For this review, take the finished solid that the model builds, in its own axes (mm). Face numbers are marked on the shaded views. A direction names the side the tool comes from. Give positions to 0.01 mm unless a question says otherwise; leave off trailing zeros. Order: outer loops, then holes, each group sorted by start corner. A loop starts at its lowest first (then second) coordinate and runs counter-clockwise, first axis right, second up. Notation, with made-up numbers: (-2, 33) - (44, 33) arc R19 ccw to (44, 55) - close; hole circle Ø7 at (-38, 33). An arc over 180 degrees is marked (long way). Use a Markdown table: item, result. Add a question column.
1) Clearance check with flat-ended pins moving along their axes: P1, Ø6, axis at x = 21, z = 28.5, coming from the +Y side; P2, Ø1.2, axis at x = -46.5, z = 11.5, coming from the -Y side; P3, Ø6, axis at x = -24.5, z = 20.5, coming from the -Y side. State where each tip first meets the part, or that it passes through.
2) We need section A-A on z = 31.5. Write out the cut boundary in (x, y).
3) Machinability: for the marked faces 1, 2 and 3, which of the approach directions +Z, -Z, +X, -X, +Y, -Y give a long, thin tool a straight path to every point of the face, cutting with its end or side? Answer none if there is none.
4) Wall thickness on L1, parallel to Z at x = 40, y = -62; L2, parallel to X at y = 25, z = 15.5: over which ranges is each line inside the solid? List them lowest first.
5) We need section B-B on x = 54. Write out the cut boundary in (y, z), then the cut area to 3 significant figures.
```python
from build123d import *

# Parameters (mm, degrees)
BOSS_EXTRU_1_DEPTH      = 2
BOSS_EXTRU_2_DEPTH      = 35
BOSS_EXTRU_3_REACH      = 144.764
BOSS_EXTRU_3_END_RADIUS = 48
ESQUISSE4_W             = 37
ESQUISSE4_H             = 2


with BuildPart() as part:
    # Esquisse1 → Boss.-Extru.1 (new body)
    with BuildSketch(Plane.XY):
        with BuildLine():
            Line((-48, 0), (-48, -68))
            Line((-48, -68), (-48, -70.5))
            Line((-48, -70.5), (70.5, -70.5))
            Line((70.5, -70.5), (70.5, -68))
            Line((70.5, -68), (70.5, 0))
            Line((70.5, 0), (68, 0))
            Line((68, 0), (48, 0))
            ThreePointArc((48, 0), (0, 48), (-48, 0))
        make_face()
    extrude(amount=BOSS_EXTRU_1_DEPTH)

    # Esquisse3 → Boss.-Extru.2 (add)
    with BuildSketch(Plane.XY.offset(2)):
        with BuildLine():
            Line((-45.5, 0), (-48, 0))
            ThreePointArc((-48, 0), (0, 48), (48, 0))
            Line((48, 0), (45.5, 0))
            ThreePointArc((45.5, 0), (0, 45.5), (-45.5, 0))
        make_face()
    extrude(amount=BOSS_EXTRU_2_DEPTH)

    # Boss.-Extru.3: up to this cylinder (the profile starts outside it)
    boss_extru_3_end = Plane(origin=(0, 0, 18.5), z_dir=(0, 0, -1)) * Cylinder(BOSS_EXTRU_3_END_RADIUS, 386.528, mode=Mode.PRIVATE)
    # Esquisse4 → Boss.-Extru.3 (add, up to the surface)
    with BuildSketch(Plane(origin=(70.5, 0, 0), x_dir=(0, 0, -1), z_dir=(1, 0, 0)), mode=Mode.PRIVATE) as boss_extru_3_sk1:
        with Locations((-18.5, 1)):
            Rectangle(ESQUISSE4_W, ESQUISSE4_H)
    boss_extru_3_tool1 = extrude(boss_extru_3_sk1.sketch, amount=-BOSS_EXTRU_3_REACH, mode=Mode.PRIVATE) - boss_extru_3_end
    add(boss_extru_3_tool1.solids().sort_by_distance((70.5, 1, 18.5))[0])


solid = part.part
```
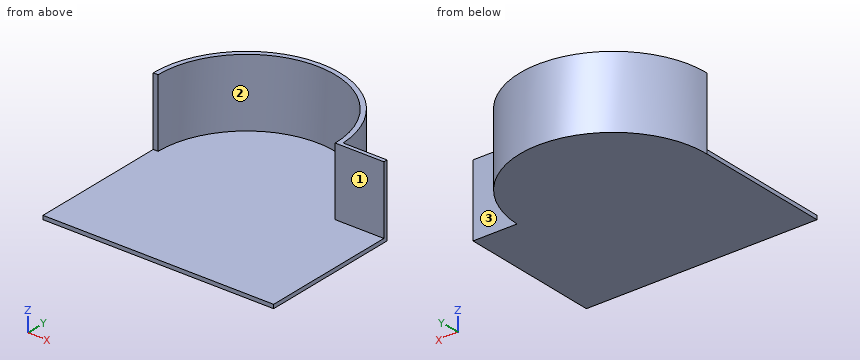
Checked values:
| question | item | result |
|---|---|---|
| 1 | P1 | y = 44.5 |
| 1 | P2 | y = 0 |
| 1 | P3 | y = 36.25 |
| 2 | outline | (-48, 0) - (-45.5, 0) arc R45.5 cw to (45.5, 0) - (70.5, 0) - (70.5, 2) - (47.96, 2) arc R48 ccw to start |
| 3 | face 1 | +Z, +X, -X, -Y |
| 3 | face 2 | +Z, -Y |
| 3 | face 3 | +Z, -Z, +X, +Y |
| 4 | L1 | 0 to 2 |
| 4 | L2 | -40.98 to -38.02, 38.02 to 40.98 |
| 5 | outline | (-70.5, 0) - (2, 0) - (2, 37) - (0, 37) - (0, 2) - (-70.5, 2) - close |
| 5 | area | 215 mm² |
